from build123d import *

# Parameters (mm, degrees)
F0_R     = 3.175
F1_DEPTH = 57.15
F2_DEPTH = 6.35
F3_R     = 0.396875


with BuildPart() as f1:
    # F0 (on Top) → F1 (new body)
    with BuildSketch(Plane.XY):
        Circle(F0_R)
    extrude(amount=F1_DEPTH)

    # F0 (on Top) → F2 (join)
    with BuildSketch(Plane.XY):
        Polygon((6.35, -3.6661742094), (6.35, 3.6661742094), (0, 7.3323484187), (-6.35, 3.6661742094), (-6.35, -3.6661742094), (0, -7.3323484187), align=None)
        Circle(F0_R, mode=Mode.SUBTRACT)
    extrude(amount=F2_DEPTH)

    # F3
    f3_edges = [f1.edges().sort_by_distance(p)[0] for p in [
        (6.35, 0, 6.35),
        (3.175, 5.499261, 6.35),
        (-3.175, 5.499261, 6.35),
        (-6.35, 0, 6.35),
        (-3.175, -5.499261, 6.35),
        (3.175, -5.499261, 6.35),
        (-3.175, 0, 6.35),
        (6.35, 0, 0),
        (3.175, 5.499261, 0),
        (-3.175, 5.499261, 0),
        (-6.35, 0, 0),
        (-3.175, -5.499261, 0),
        (3.175, -5.499261, 0),
        (-3.175, 0, 57.15),
    ]]
    fillet(f3_edges, radius=F3_R)


solid = f1.part
Source: CAD feature listing. Evaluate the final solid. Frame: model axes, mm. A direction names the side the tool comes from. Round coordinates to 2 decimals unless told otherwise and drop trailing zeros. Loops run counter-clockwise (first coordinate to the right, second up) from the corner with the lowest first, then second, coordinate; pieces in that order, holes last. Notation, with made-up numbers: M 67,45.5 L 92,45.5 A19 ccw 92,64.5 Z; hole C 56,80 d8. An arc over 180 degrees is marked long. Return JSON: item names as keys, results as strings. Group by question number.
1. Pin query (flat end, axial travel): pin 1 (1.5 mm diameter, centred on x = 1, z = 6, fed in from +Y); pin 2 (1 mm diameter, centred on x = 3, z = 13.5, fed in from -Y); pin 3 (6 mm diameter, centred on x = 1.5, z = 27.5, fed in from -Y) (3 decimals). Return the tip coordinate at first contact, or that it passes through.
2. Section query A-A on y = 0. Output: boundary loops of the cut face in (x, z) (3 decimals).
3. Material intervals for line 1 along Z through (x, y) = (3.75, -1.5); line 2 along X through (y, z) = (-3.5, 6); line 3 along Z through (x, y) = (-5.25, 4.25), sorted ascending. Write a range as from..to.
4. Reachability of faces 1 (the face through (3.131, -5.525, 3.136)), 2 (the face through (-0.69, -3.1, 31.4)) from +Z, -Z, +X, -X, +Y, -Y: full face, straight path, thin tool, end or side. Return the list, or none.
5. Section query B-B on z = 43.5. Output: boundary loops of the cut face in (x, y) (3 decimals).
Checks:
{
 "1": {"pin 1": "stops at y = 7.19", "pin 2": "stops at y = -1.96", "pin 3": "stops at y = -3.175"},
 "2": {"outline": "M -6.35,0.397 A0.397 ccw -5.953,0 L 5.953,0 A0.397 ccw 6.35,0.397 L 6.35,5.953 A0.397 ccw 5.953,6.35 L 3.572,6.35 A0.397 cw 3.175,6.747 L 3.175,56.753 A0.397 ccw 2.778,57.15 L -2.778,57.15 A0.397 ccw -3.175,56.753 L -3.175,6.747 A0.397 cw -3.572,6.35 L -5.953,6.35 A0.397 ccw -6.35,5.953 Z"},
 "3": {"line 1": "z = 0..6.35", "line 2": "x = -6.35..6.35", "line 3": "z = 0.21..6.14"},
 "4": {"face 1": "+Z, -Z, +X, -Y", "face 2": "+Z"},
 "5": {"outline": "C 0,0 d6.35"}
}
